Source: CAD feature listing. Evaluate the final solid. Frame: model axes, mm. Face numbers are marked on the shaded views. A direction names the side the tool comes from. Round coordinates to 2 decimals unless told otherwise and drop trailing zeros. Write each loop counter-clockwise with the first axis right and the second up, starting at its lowest first coordinate (ties: lowest second). Pieces come first, ordered by that corner, then holes. Notation, with made-up numbers: M 14,72 L 46,72 A10 ccw 46,78 Z; hole C 16,-24.75 d8. An arc over 180 degrees is marked long. Answer in a Markdown table with one row per item.
from build123d import *

# Parameters (mm, degrees)
BOSS_EXTRU_1_DEPTH = 50
BOSS_EXTRU_2_DEPTH = 50
BOSS_EXTRU_3_DEPTH = 50


with BuildPart() as part:
    # Esquisse1 → Boss.-Extru.1 (new body)
    with BuildSketch(Plane.XY):
        Polygon((-40, 100), (-70, 100), (-70, 70), (0, 70), (0, 0), (-20, 0), (-20, 50), (-95, 50), (-95, 120), (-40, 120), align=None)
    extrude(amount=-BOSS_EXTRU_1_DEPTH)

    # Esquisse3 → Boss.-Extru.2 (add)
    with BuildSketch(Plane.XY):
        Polygon((-45, 50), (-20, 40), (-20, 50), align=None)
    extrude(amount=-BOSS_EXTRU_2_DEPTH)

    # Esquisse3<4> → Boss.-Extru.3 (add)
    with BuildSketch(Plane.XY):
        Polygon((-70, 100), (-70, 85), (-55, 100), align=None)
    extrude(amount=-BOSS_EXTRU_3_DEPTH)


solid = part.part
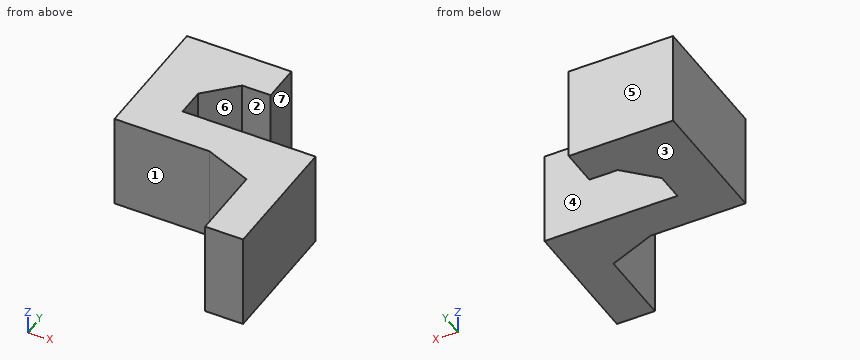
Q1. Material intervals for probe 1 along Y at (x, z) = (-78.5, -42); probe 2 along X at (y, z) = (27.5, -41); probe 3 along X at (y, z) = (104.5, -42.5), sorted ascending.
Solutions:
| item | result |
|---|---|
| probe 1 | y = 50 to 120 |
| probe 2 | x = -20 to 0 |
| probe 3 | x = -95 to -40 |
Q2. Pull-direction query (Y, two-part tool) for the marked faces 4, 5, 6 and 7; classes: pulls with the +Y half, pulls with the -Y half, needs draft (parallel to the pull), parting line crosses it, or undercut.
Solutions:
| item | result |
|---|---|
| face 4 | undercut |
| face 5 | pulls with the +Y half |
| face 6 | undercut |
| face 7 | needs draft |
Q3. Section D-D (y = 81). Return loops of the section in (x, z).
Solutions:
| item | result |
|---|---|
| outline | M -95,-50 L -70,-50 L -70,0 L -95,0 Z |
Q4. Contact query for flat-ended pins moving along their axis: pin 1 Ø20 at (y, z) = (18.5, -36) entering from -X; pin 2 Ø6 at (x, z) = (-18.5, -15) entering from +Y; pin 3 Ø4.5 at (x, z) = (-49.5, -24.5) entering from -Y. Output: stop coordinate, or through.
Solutions:
| item | result |
|---|---|
| pin 1 | stops at x = -20 |
| pin 2 | stops at y = 70 |
| pin 3 | stops at y = 50 |
Q5. Access query for the marked faces 1, 2 and 3. Directions: +Z, -Z, +X, -X, +Y, -Y. A direction counts if a zero-diameter tool reaches every point of the face in a straight line with its end or side. Return the directions, or none.
Solutions:
| item | result |
|---|---|
| face 1 | +Z, -Z, -X, -Y |
| face 2 | +Z, -Z, +X |
| face 3 | -Z, +X, -X, +Y, -Y |
Q6. Section B-B (z = -14.5). Return loops of the section in (x, y).
Solutions:
| item | result |
|---|---|
| outline | M -95,50 L -45,50 L -20,40 L -20,0 L 0,0 L 0,70 L -70,70 L -70,85 L -55,100 L -40,100 L -40,120 L -95,120 Z |
Q7. Section A-A (x = -65). Return loops of the section in (y, z), and give its area (3 significant figures).
Solutions:
| item | result |
|---|---|
| outline | M 50,-50 L 70,-50 L 70,0 L 50,0 Z; M 90,-50 L 120,-50 L 120,0 L 90,0 Z |
| area | 2,500 mm2 |
Q8. Section C-C (x = -47). Return loops of the section in (y, z), and give its area (3 significant figures).
Solutions:
| item | result |
|---|---|
| outline | M 50,-50 L 70,-50 L 70,0 L 50,0 Z; M 100,-50 L 120,-50 L 120,0 L 100,0 Z |
| area | 2,000 mm2 |
